Design review of the part built by this model. Coordinates are the model's own, in mm. Face numbers are marked on the shaded views. A direction names the side the tool comes from. Round coordinates to 2 decimals unless told otherwise and drop trailing zeros. Write each loop counter-clockwise with the first axis right and the second up, starting at its lowest first coordinate (ties: lowest second). Pieces come first, ordered by that corner, then holes. Notation, with made-up numbers: (-29, 43.25) -> (11, 43.25) arc R30 ccw to (11, 66.25) -> close; hole circle Ø6 at (-13.75, 86). An arc over 180 degrees is marked (long way). One line per question, with ' | ' between items. Start each with the question number.
1) Consider section C-C (x = -3.75). Give the boundary of the cut face in (y, z).
2) For the marked faces 1, 2 and 3, list the 3-axis set-ups (+Z, -Z, +X, -X, +Y, -Y) from which the entire face can be reached by the end or side of a thin tool; tool diameter is ignored.
3) Consider section B-B (z = -9.5). Give the boundary of the cut face in (x, y), then the cut area to 3 significant figures.
4) Insertion check: pin 1 Ø2 at (y, z) = (-4.5, -16) entering from -X; pin 2 Ø4 at (x, y) = (9.5, 0.5) entering from +Z; pin 3 Ø0.5 at (y, z) = (5.5, -1) entering from +X; pin 4 Ø0.6 at (y, z) = (5.5, -8.5) entering from -X. Each pin has a flat end and moves straight along its axis. Give the tip position at first contact, or say it passes through.
5) Mouldability with a two-part tool opening along Y and no side actions: class the marked faces 4, 5, 6 and 7 as +Y half, -Y half, draft (parallel to the pull), parting line (faces both ways), or undercut.
6) Consider section D-D (x = 3.5). Give the boundary of the cut face in (y, z).
7) For probe 1 along Z at (x, y) = (16, -4.5); probe 2 along Y at (x, z) = (0, -0.6); probe 3 along Z at (x, y) = (6.25, 3.5), list the stretches that pass through material, from the lowest coordinate up.
8) Consider section A-A (y = 0). Count the separate pieces of the cut face and the enclosed holes in it, then the cut area to 3 significant figures.
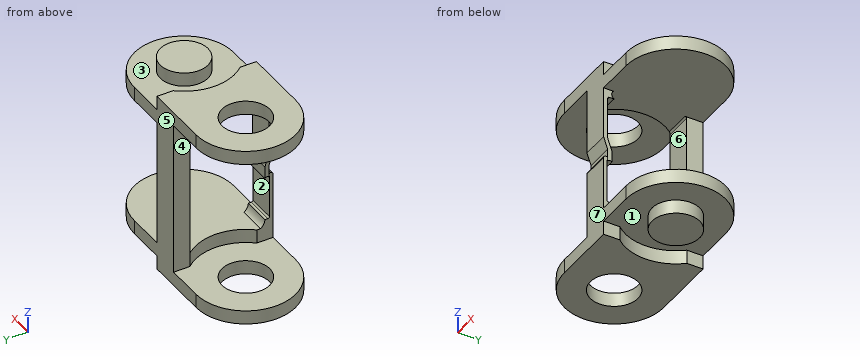
Autodesk Inventor part; units mm, degrees
ref_plane "R1_XY" through (0, 0, 0) normal (0, 0, 1) x (1, 0, 0)
ref_plane "R1_YZ" through (0, 0, 0) normal (1, 0, 0) x (0, 1, 0)
ref_plane "R1_ZX" through (0, 0, 0) normal (0, 1, 0) x (0, 0, 1)
sketch "Sketch_1" plane through (0, 0, 0) normal (0, 0, 1) x (1, 0, 0)
  arc A0 (0, 6.25) -> (0, -6.25) centre (0, 0) ccw
  line L0 (0, -6.25) -> (8.25, -6.25)
  line L1 (8.25, -6.25) -> (8.25, -4.2143)
  arc A1 (8.25, 4.2143) -> (8.25, -4.2143) centre (13, 0) ccw
  line L2 (8.25, 4.2143) -> (8.25, 6.25)
  line L3 (8.25, 6.25) -> (0, 6.25)
  circle A2 centre (0, 0) radius 3
extrude "Extrusion1" add sketch "Sketch_1" against normal blind 1.75
sketch "Sketch_3" plane through (0, 0, -1.75) normal (0, 0, 1) x (1, 0, 0)
  circle A0 centre (13, 0) radius 3
sketch "Sketch_6" plane through (0, 0, -21.25) normal (0, 0, 1) x (1, 0, 0)
  circle A0 centre (13, 0) radius 3
sketch "Sketch_7" plane through (0, 0, -21.25) normal (0, 0, 1) x (1, 0, 0)
  arc A0 (0, 6.25) -> (0, -6.25) centre (0, 0) ccw
  line L0 (0, -6.25) -> (8.25, -6.25)
  line L1 (8.25, -6.25) -> (8.25, -4.2143)
  arc A1 (8.25, 4.2143) -> (8.25, -4.2143) centre (13, 0) ccw
  line L2 (8.25, 4.2143) -> (8.25, 6.25)
  line L3 (8.25, 6.25) -> (0, 6.25)
  circle A2 centre (0, 0) radius 3
sketch "Sketch_4" plane through (0, 0, -19.5) normal (0, 0, 1) x (1, 0, 0)
  line L0 (4.75, 6.25) -> (4.75, -6.25)
  line L1 (4.75, -6.25) -> (13, -6.25)
  arc A0 (13, -6.25) -> (13, 6.25) centre (13, 0) ccw
  line L2 (13, 6.25) -> (4.75, 6.25)
sketch "Sketch_5" plane through (0, 0, -1.75) normal (0, 0, 1) x (1, 0, 0)
  line L0 (4.75, 6.25) -> (4.75, -6.25)
  line L1 (4.75, -6.25) -> (13, -6.25)
  arc A0 (13, -6.25) -> (13, 6.25) centre (13, 0) ccw
  line L2 (13, 6.25) -> (4.75, 6.25)
extrude "Extrusion2" add sketch "Sketch_5" against normal blind 1.75
extrude "Extrusion3" add sketch "Sketch_3" along normal blind 1.75
sketch "Sketch_9" plane through (6.5, 0, 0) normal (1, 0, 0) x (0, 0, -1)
  arc A0 (3.7, 4.173) -> (3.5, 3.973) centre (3.7, 3.973) ccw
  line L0 (3.7, 4.173) -> (19.3, 4.173)
  arc A1 (19.5, 3.973) -> (19.3, 4.173) centre (19.3, 3.973) ccw
  line L1 (19.5, 3.973) -> (19.5, 6.25)
  line L2 (19.5, 6.25) -> (3.5, 6.25)
  line L3 (3.5, 6.25) -> (3.5, 3.973)
extrude "Extrusion4" add sketch "Sketch_9" along normal mid plane 3.5
sketch "Sketch_11" plane through (6.5, 0, 0) normal (1, 0, 0) x (0, 0, -1)
  line L0 (3.5, -5.0148) -> (3.5, -6.25)
  line L1 (3.5, -6.25) -> (10, -6.25)
  line L2 (10, -6.25) -> (11.5, -5.7333)
  line L3 (11.5, -5.7333) -> (13, -5.7333)
  arc A0 (13, -5.2167) -> (13, -5.7333) centre (13.2583, -5.475) ccw
  line L4 (13, -5.2167) -> (11.5, -5.2167)
  line L5 (11.5, -5.2167) -> (10, -5.7333)
  line L6 (10, -5.7333) -> (4.7, -5.7333)
  arc A1 (4.5, -5.5333) -> (4.7, -5.7333) centre (4.7, -5.5333) ccw
  line L7 (4.5, -5.5333) -> (4.5, -4.9347)
  arc A2 (3.5, -5.0148) -> (4.5, -4.9347) centre (3.97, -4.6003) ccw
extrude "Extrusion5" add sketch "Sketch_11" along normal mid plane 3.5
sketch "Sketch_12" plane through (6.5, 0, 0) normal (1, 0, 0) x (0, 0, -1)
  line L0 (12.5, -5.8071) -> (12.5, -5.95)
  arc A0 (12.5, -5.95) -> (12.8, -6.25) centre (12.8, -5.95) ccw
  line L1 (12.8, -6.25) -> (19.5, -6.25)
  line L2 (19.5, -6.25) -> (19.5, -4.6689)
  arc A1 (18.5, -5.227) -> (19.5, -4.6689) centre (18.5, -4.052) ccw
  line L3 (18.5, -5.227) -> (18.5, -5.6071)
  arc A2 (18.3, -5.8071) -> (18.5, -5.6071) centre (18.3, -5.6071) ccw
  line L4 (18.3, -5.8071) -> (13.049, -5.8071)
  arc A3 (12.9618, -5.7915) -> (13.049, -5.8071) centre (13.049, -5.5571) ccw
  arc A4 (12.9618, -5.7915) -> (12.5, -5.8071) centre (12.75, -6.361) ccw
extrude "Extrusion6" add sketch "Sketch_4" against normal blind 1.75
extrude "Extrusion7" add sketch "Sketch_6" against normal blind 1.75
extrude "Extrusion8" add sketch "Sketch_7" against normal blind 1.75
extrude "Extrusion9" add sketch "Sketch_12" along normal mid plane 3.5
sketch "Sketch_19" plane through (0, 0, -1.75) normal (0, 0, 1) x (1, 0, 0)
  line L0 (-8.25, 6.35) -> (-8.25, -6.35)
  line L1 (-8.25, -6.35) -> (0, -6.35)
  arc A0 (0, -6.35) -> (0, 6.35) centre (0, 0) ccw
  line L2 (0, 6.35) -> (-8.25, 6.35)
extrude "Extrusion10" cut sketch "Sketch_19" against normal blind 9.75
sketch "Sketch_20" plane through (0, 0, -21.25) normal (0, 0, 1) x (1, 0, 0)
  line L0 (-8.25, 6.35) -> (-8.25, -6.35)
  line L1 (-8.25, -6.35) -> (0, -6.35)
  arc A0 (0, -6.35) -> (0, 6.35) centre (0, 0) ccw
  line L2 (0, 6.35) -> (-8.25, 6.35)
extrude "Extrusion11" cut sketch "Sketch_20" along normal blind 9.75
ref_plane "R1_XY" through (0, 0, 0) normal (0, 0, 1) x (1, 0, 0)
ref_plane "R1_YZ" through (0, 0, 0) normal (1, 0, 0) x (0, 1, 0)
ref_plane "R1_ZX" through (0, 0, 0) normal (0, 1, 0) x (0, 0, 1)
ref_plane "clip_to_dummy_XY" through (6.5, -18, -11.5) normal (0, 0, 1) x (1, 0, 0)
ref_plane "clip_to_dummy_YZ" through (6.5, -18, -11.5) normal (1, 0, 0) x (0, 1, 0)
ref_plane "clip_to_dummy_ZX" through (6.5, -18, -11.5) normal (0, 1, 0) x (0, 0, 1)
ref_plane "move_1_XY" through (13, 0, 0) normal (0, 0, 1) x (1, 0, 0)
ref_plane "move_1_YZ" through (13, 0, 0) normal (1, 0, 0) x (0, 1, 0)
ref_plane "move_1_ZX" through (13, 0, 0) normal (0, 1, 0) x (0, 0, 1)
ref_plane "move_2_XY" through (0, 0, 0) normal (0, 0, 1) x (1, 0, 0)
ref_plane "move_2_YZ" through (0, 0, 0) normal (1, 0, 0) x (0, 1, 0)
ref_plane "move_2_ZX" through (0, 0, 0) normal (0, 1, 0) x (0, 0, 1)
ref_plane "move_end_XY" through (13, 0, 0) normal (0, 0, 1) x (1, 0, 0)
ref_plane "move_end_YZ" through (13, 0, 0) normal (1, 0, 0) x (0, 1, 0)
ref_plane "move_end_ZX" through (13, 0, 0) normal (0, 1, 0) x (0, 0, 1)
properties part number "SZ045F-16-018-27c"
From the geometry:
1) outline: (-5, -23) -> (5, -23) -> (5, -21.25) -> (-5, -21.25) -> close; (-5, -1.75) -> (5, -1.75) -> (5, 0) -> (-5, 0) -> close
2) face 1: -Z | face 2: +X, -X | face 3: +Z
3) outline: (4.75, -6.25) -> (8.25, -6.25) -> (8.25, -5.73) -> (4.75, -5.73) -> close; (4.75, 4.21) arc R6.35 cw to (4.79, 4.17) -> (8.25, 4.17) -> (8.25, 6.25) -> (4.75, 6.25) -> close | area: 9.08 mm2
4) pin 1: passes through | pin 2: stops at z = 0 | pin 3: stops at x = 8.25 | pin 4: stops at x = 4.75
5) face 4: draft | face 5: +Y half | face 6: undercut | face 7: -Y half
6) outline: (-6.25, -23) -> (6.25, -23) -> (6.25, -21.25) -> (-6.25, -21.25) -> close; (-6.25, -1.75) -> (6.25, -1.75) -> (6.25, 0) -> (-6.25, 0) -> close
7) probe 1: z = -21.25 to -19.5, -3.5 to -1.75 | probe 2: y = -6.25 to -3, 3 to 6.25 | probe 3: z = -23 to -19.5, -3.5 to 0
8) separate pieces: 4 | enclosed holes: 0 | area: 90.3 mm2
